```python
from build123d import *

# Parameters (mm, degrees)
SKETCH1_W                 = 130.000000096
SKETCH1_H                 = 43.000000106
BOSS_EXTRUDE1_DEPTH       = 42.999999979
M3X0_5_TAPPED_HOLE1_D     = 2.5
M3X0_5_TAPPED_HOLE1_DEPTH = 1.999996
M3X0_5_TAPPED_HOLE1_TIP   = 0.751075774
SKETCH4_R                 = 12.7
CUT_EXTRUDE1_DEPTH        = 2.54


with BuildPart() as part:
    # Sketch1 → Boss-Extrude1 (new, symmetric)
    with BuildSketch(Plane.XY):
        Rectangle(SKETCH1_W, SKETCH1_H)
    extrude(amount=BOSS_EXTRUDE1_DEPTH, both=True)

    # M3x0.5 Tapped Hole1
    with Locations(Plane(origin=(0, -21.500000053, 0), x_dir=(-1, 0, 0), z_dir=(0, -1, 0))):
        with Locations((60.000000142, -24.700000003), (-60.000000142, -24.700000003), (-60.000000142, 25.300000073), (60.000000142, 25.300000073)):
            Hole(M3X0_5_TAPPED_HOLE1_D / 2, depth=M3X0_5_TAPPED_HOLE1_DEPTH)
            with Locations((0, 0, -(M3X0_5_TAPPED_HOLE1_DEPTH + M3X0_5_TAPPED_HOLE1_TIP / 2))):  # 118° drill point
                Cone(0, M3X0_5_TAPPED_HOLE1_D / 2, M3X0_5_TAPPED_HOLE1_TIP, mode=Mode.SUBTRACT)

    # Sketch4 → Cut-Extrude1 (cut)
    with BuildSketch(Plane(origin=(0, 0, -42.999999979), x_dir=(-1, 0, 0), z_dir=(0, 0, -1))):
        Circle(SKETCH4_R)
    extrude(amount=-CUT_EXTRUDE1_DEPTH, mode=Mode.SUBTRACT)


solid = part.part
```
Check sheet for the modelled part. Datum: model origin and axes. Units: mm. A direction names the side the tool comes from. Round coordinates to 2 decimals unless told otherwise and drop trailing zeros. Loops run counter-clockwise (first coordinate to the right, second up) from the corner with the lowest first, then second, coordinate; pieces in that order, holes last. Notation, with made-up numbers: (-1, -27) - (50, -27) arc R12 ccw to (50, -6) - close; hole circle Ø11 at (68.5, -3). An arc over 180 degrees is marked (long way). Answer as a JSON object with one key per item and string values. Group by question number.
Q1. Mould release check, pull along Z, two halves, no side actions. Record for faces 4 (the face through (-1, -21.5, 1)), 5 (the face through (-1, 0, 43)), 6 (the face through (-60.2, -18.88, 24.78)): released by +Z, released by -Z, zero draft, split by the parting line, or undercut.
Q2. Sectioned sample at A-A, the plane x = 0. Enter the section's corners in (y, z), plus the area to 3 significant figures.
Q3. Scan lines: line 1 along Z through (x, y) = (-60, -20); line 2 along X through (y, z) = (-20, 24); line 3 along X through (y, z) = (-20, -25). Record each from-to range of solid material in increasing order. Write a range as [from, to].
Q4. Set-up check for faces 1 (the face through (-1, 21.5, 1)), 2 (the face through (0, 0, -40.46)), 3 (the face through (-59.423, -20.486, 25.809)): record each of +Z, -Z, +X, -X, +Y, -Y from which the full face is reachable in a straight line by a thin tool's end or side.
Q5. Gauge pin test, flat end, axial feed: P1, Ø20.5, axis at x = 0, y = 0, coming from the -Z side. Record the tip position at first contact, or that the pin passes through.
Solution:
{
 "1": {"face 4": "zero draft", "face 5": "released by +Z", "face 6": "undercut"},
 "2": {"outline": "(-21.5, -43) - (-12.7, -43) - (-12.7, -40.46) - (12.7, -40.46) - (12.7, -43) - (21.5, -43) - (21.5, 43) - (-21.5, 43) - close", "area": "3,630 mm²"},
 "3": {"line 1": "z = [-43, -26.55], [-24.05, 23.45], [25.95, 43]", "line 2": "x = [-65, -61.04], [-58.96, 58.96], [61.04, 65]", "line 3": "x = [-65, -61.21], [-58.79, 58.79], [61.21, 65]"},
 "4": {"face 1": "+Z, -Z, +X, -X, +Y", "face 2": "-Z", "face 3": "-Y"},
 "5": {"P1": "stops at z = -40.46"}
}
